Design review of the part shown in the three views and the two pictorial views. Dimensions are in mm from the part's minimum x, y and z. A direction names the side the tool comes from. Round coordinates to 2 decimals unless told otherwise and drop trailing zeros. Order: outer loops, then holes, each group sorted by start corner. A loop starts at its lowest first (then second) coordinate and runs counter-clockwise, first axis right, second up. Notation, with made-up numbers: (21, 73.5) - (78, 73.5) arc R24 cw to (78, 94.5) - close; hole circle Ø8 at (44, 71). An arc over 180 degrees is marked (long way). Use CSV: the item, a comma, the result in double quotes.
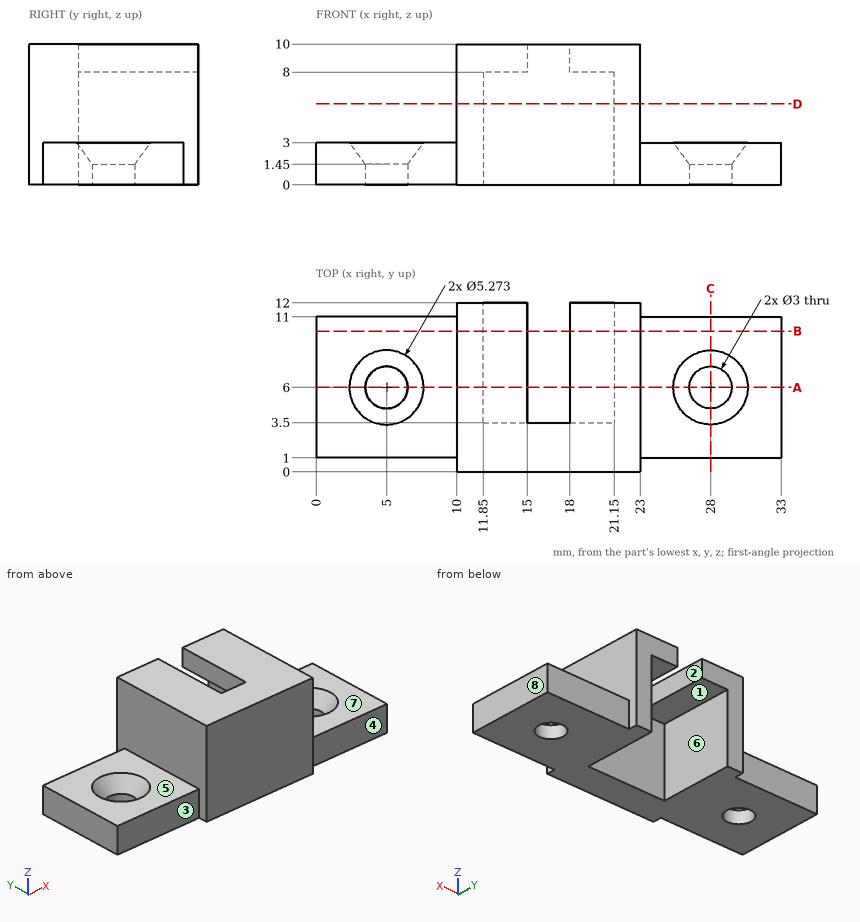
1) Insertion check: pin 1 Ø2 at (y, z) = (6.5, 9.5) entering from +X; pin 2 Ø4.5 at (x, z) = (18.5, 6.5) entering from +Y; pin 3 Ø3.5 at (x, y) = (28, 6) entering from +Z; pin 4 Ø3.5 at (x, z) = (7.5, 1.5) entering from -Y. Each pin has a flat end and moves straight along its axis. Give the tip position at first contact, or say it passes through.
Data:
pin 1,"stops at x = 23"
pin 2,"stops at y = 12"
pin 3,"stops at z = 1.79"
pin 4,"stops at y = 1"
2) For the marked faces 1, 2, 3, 4 and 5, list the 3-axis set-ups (+Z, -Z, +X, -X, +Y, -Y) from which the entire face can be reached by the end or side of a thin tool; tool diameter is ignored.
Data:
face 1,"-Z, +Y"
face 2,"+Z, -Z, +Y"
face 3,"+Z, -Z, -X, -Y"
face 4,"+Z, -Z, +X, -Y"
face 5,"+Z, -X, +Y, -Y"
3) We need section A-A (y = 6). Give the boundary of the cut face in (x, z).
Data:
outline,"(0, 0) - (3.5, 0) - (3.5, 1.45) - (2.36, 3) - (0, 3) - close; (6.5, 0) - (11.85, 0) - (11.85, 8) - (15, 8) - (15, 10) - (10, 10) - (10, 3) - (7.64, 3) - (6.5, 1.45) - close; (18, 8) - (21.15, 8) - (21.15, 0) - (26.5, 0) - (26.5, 1.45) - (25.36, 3) - (23, 3) - (23, 10) - (18, 10) - close; (29.5, 0) - (33, 0) - (33, 3) - (30.64, 3) - (29.5, 1.45) - close"
4) We need section C-C (x = 28). Give the boundary of the cut face in (y, z).
Data:
outline,"(1, 0) - (4.5, 0) - (4.5, 1.45) - (3.36, 3) - (1, 3) - close; (7.5, 0) - (11, 0) - (11, 3) - (8.64, 3) - (7.5, 1.45) - close"
5) The part is to be moulded in two halves that separate along X. For the marked faces 6, 7 and 8, say which applies: +X half, -X half, draft (parallel to the pull), parting line (faces both ways), or undercut.
Data:
face 6,"undercut"
face 7,"draft"
face 8,"+X half"
6) To check wall thickness, follow L1, parallel to X at y = 6, z = 0.65; L2, parallel to X at y = 3.75, z = 5.25; L3, parallel to Y at x = 5, z = 1.1. State the ranges of each line that lie inside material, in increasing order. Write a range as from..to.
Data:
L1,"x = 0..3.5, 6.5..11.85, 21.15..26.5, 29.5..33"
L2,"x = 10..11.85, 21.15..23"
L3,"y = 1..4.5, 7.5..11"
7) We need section D-D (z = 5.75). Give the boundary of the cut face in (x, y).
Data:
outline,"(10, 0) - (23, 0) - (23, 12) - (21.15, 12) - (21.15, 3.5) - (11.85, 3.5) - (11.85, 12) - (10, 12) - close"
8) We need section B-B (y = 10). Give the boundary of the cut face in (x, z), then the cut area to 3 significant figures.
Data:
outline,"(0, 0) - (11.85, 0) - (11.85, 8) - (15, 8) - (15, 10) - (10, 10) - (10, 3) - (0, 3) - close; (18, 8) - (21.15, 8) - (21.15, 0) - (33, 0) - (33, 3) - (23, 3) - (23, 10) - (18, 10) - close"
area,"110 mm2"
